```python
from build123d import *

# Parameters (mm, degrees)
SKETCH_1_R      = 1
EXTRUDE_1_DEPTH = 1.5


with BuildPart() as part:
    # 草图1 → 凸台-拉伸1 (new body)
    with BuildSketch(Plane.XY):
        Polygon((-19.000504276, 4), (18.999495724, 4), (18.999495724, 2), (20.5, 2), (20.5, 3.7), (22.499555553, 3.7), (22.499555553, 2), (24.00005983, 2), (24.00005983, 3.7), (25.999615383, 3.7), (25.999615383, 2), (27.50011966, 2), (27.50011966, 4), (29.499675213, 4), (29.499675213, -3.6), (27.5, -3.6), (27.5, -1.6), (26, -1.6), (26, -3.3), (24, -3.3), (24, -1.6), (22.5, -1.6), (22.5, -3.3), (20.5, -3.3), (20.5, -1.6), (19, -1.6), (19, -3.6), (-19, -3.6), (-19, -1.6), (-20.5, -1.6), (-20.5, -3.3), (-22.5, -3.3), (-22.5, -1.6), (-24, -1.6), (-24, -3.3), (-26, -3.3), (-26, -1.6), (-27.5, -1.6), (-27.5, -3.6), (-29.5, -3.6), (-29.5, 4.4), (-27.5, 4.4), (-27.5, 2.2), (-26, 2.2), (-26, 3.9), (-24, 3.9), (-24, 2.2), (-22.5, 2.2), (-22.5, 3.9), (-20.5, 3.9), (-20.5, 2.2), (-19.000504276, 2.2), align=None)
        Circle(SKETCH_1_R, mode=Mode.SUBTRACT)
        with Locations((5, 0)):
            Circle(SKETCH_1_R, mode=Mode.SUBTRACT)
        with Locations((10, 0)):
            Circle(SKETCH_1_R, mode=Mode.SUBTRACT)
        with Locations((15, 0)):
            Circle(SKETCH_1_R, mode=Mode.SUBTRACT)
        with Locations((-5, 0)):
            Circle(SKETCH_1_R, mode=Mode.SUBTRACT)
        with Locations((-10, 0)):
            Circle(SKETCH_1_R, mode=Mode.SUBTRACT)
        with Locations((-15, 0)):
            Circle(SKETCH_1_R, mode=Mode.SUBTRACT)
    extrude(amount=EXTRUDE_1_DEPTH)


solid = part.part
```
The model under review builds one solid part; all positions refer to its coordinate system, in mm. A direction names the side the tool comes from. Round coordinates to 2 decimals unless told otherwise and drop trailing zeros. Order: outer loops, then holes, each group sorted by start corner. A loop starts at its lowest first (then second) coordinate and runs counter-clockwise, first axis right, second up. Notation, with made-up numbers: (-33.75, 45.5) - (-28.75, 45.5) arc R16 cw to (-28.75, 64.5) - close; hole circle Ø2 at (67.25, -7). An arc over 180 degrees is marked (long way). Answer in a Markdown table with one row per item.
(1) For line 1 (X direction, y = 3.75, z = 1.3); line 2 (Y direction, x = 10, z = 0.9); line 3 (Y direction, x = -2, z = 0.8), list the stretches that pass through material, from the lowest coordinate up. Write a range as from..to.
Result set:
| item | result |
|---|---|
| line 1 | x = -29.5..-27.5, -26..-24, -22.5..-20.5, -19..19, 27.5..29.5 |
| line 2 | y = -3.6..-1, 1..4 |
| line 3 | y = -3.6..4 |
(2) Clearance check with flat-ended pins moving along their axes: P1, Ø0.8, axis at x = 22, z = 1, coming from the -Y side; P2, Ø0.8, axis at x = 23, z = 0.5, coming from the -Y side. State where each tip first meets the part, or that it passes through.
Result set:
| item | result |
|---|---|
| P1 | stops at y = -3.3 |
| P2 | stops at y = -1.6 |
(3) Take a section at C-C on y = 3. Write out the cut boundary in (x, z), plus the area to 3 significant figures.
Result set:
| item | result |
|---|---|
| outline | (-29.5, 0) - (-27.5, 0) - (-27.5, 1.5) - (-29.5, 1.5) - close; (-26, 0) - (-24, 0) - (-24, 1.5) - (-26, 1.5) - close; (-22.5, 0) - (-20.5, 0) - (-20.5, 1.5) - (-22.5, 1.5) - close; (-19, 0) - (19, 0) - (19, 1.5) - (-19, 1.5) - close; (20.5, 0) - (22.5, 0) - (22.5, 1.5) - (20.5, 1.5) - close; (24, 0) - (26, 0) - (26, 1.5) - (24, 1.5) - close; (27.5, 0) - (29.5, 0) - (29.5, 1.5) - (27.5, 1.5) - close |
| area | 75.0 mm2 |
(4) Machinability: for faces 3 (the face through (9.2, -0.6, 0.7)), 4 (the face through (-20.5, -2, 1)), 5 (the face through (-25, 3.9, 1)), which of the approach directions +Z, -Z, +X, -X, +Y, -Y give a long, thin tool a straight path to every point of the face, cutting with its end or side? Answer none if there is none.
Result set:
| item | result |
|---|---|
| face 3 | +Z, -Z |
| face 4 | +Z, -Z, -Y |
| face 5 | +Z, -Z, +Y |
(5) Take a section at A-A on y = 0. Count the separate pieces of the cut face and the enclosed holes in it, plus the area to 3 significant figures.
Result set:
| item | result |
|---|---|
| separate pieces | 8 |
| enclosed holes | 0 |
| area | 67.5 mm2 |
(6) Mouldability with a two-part tool opening along X and no side actions: class faces 1 (the face through (-28, -3.6, 1)), 2 (the face through (-27, 2.2, 1)) as released by +X, released by -X, zero draft, split by the parting line, or undercut.
Result set:
| item | result |
|---|---|
| face 1 | zero draft |
| face 2 | undercut |
(7) Take a section at B-B on x = 5. Write out the cut boundary in (y, z), plus the area to 3 significant figures.
Result set:
| item | result |
|---|---|
| outline | (-3.6, 0) - (-1, 0) - (-1, 1.5) - (-3.6, 1.5) - close; (1, 0) - (4, 0) - (4, 1.5) - (1, 1.5) - close |
| area | 8.40 mm2 |
